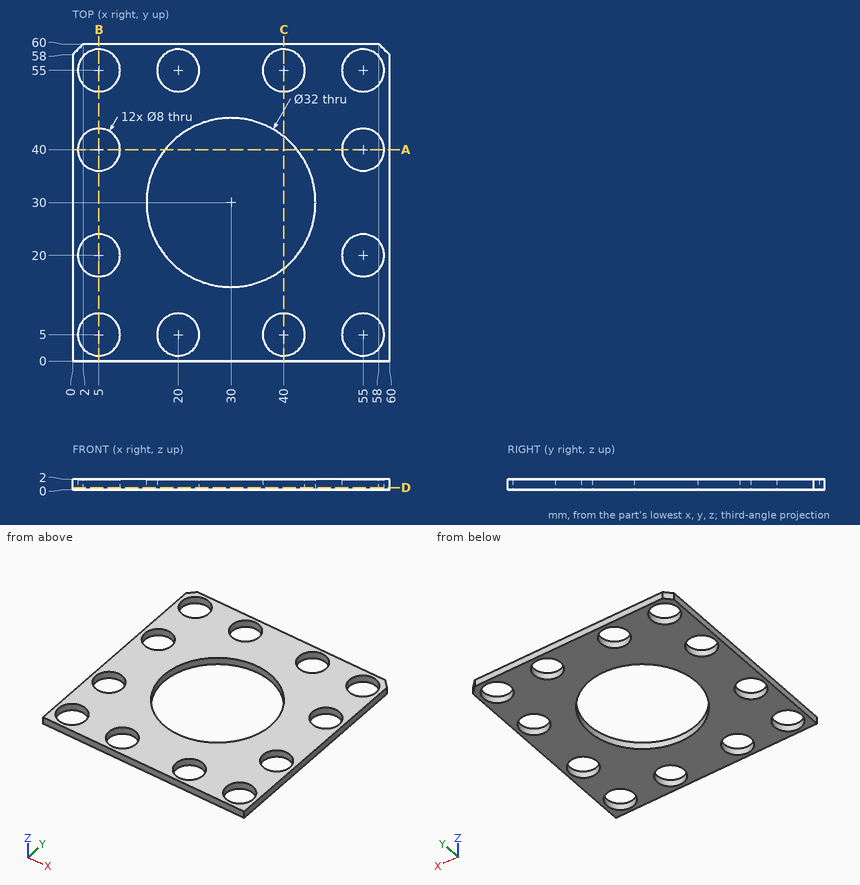
Study the drawing (mm; zero at the part's minimum x, y, z) and answer. Round coordinates to 2 decimals unless told otherwise and drop trailing zeros. Loops run counter-clockwise (first coordinate to the right, second up) from the corner with the lowest first, then second, coordinate; pieces in that order, holes last. Notation, with made-up numbers: (32.5, -1.5) -> (50.5, -1.5) arc R18 cw to (50.5, 23.5) -> close; hole circle Ø2 at (-31, 30.5). An arc over 180 degrees is marked (long way). Write each question's results on one line, items separated by ' | '. Start each with the question number.
1. Section A-A (y = 40) is taken. Determine the outline of the cut face in (x, z).
2. Section D-D (z = 0.35) is taken. State how many separate pieces and enclosed holes the cut face has, plus the area to 3 significant figures.
3. Given pin 1 Ø5 at (x, y) = (40, 5) entering from -Z, flat-ended and moving along its own axis, determine where the tip first touches the part or whether it passes through.
4. Find the intervals of material crossed by probe 1 along Y at (x, z) = (55, 1.25); probe 2 along Y at (x, z) = (21.5, 0.95); probe 3 along Y at (x, z) = (8, 1.25), in increasing order. Write a range as from..to.
5. Section B-B (x = 5) is taken. Determine the outline of the cut face in (y, z).
Evaluation:
1) outline: (0, 0) -> (1, 0) -> (1, 2) -> (0, 2) -> close; (9, 0) -> (17.51, 0) -> (17.51, 2) -> (9, 2) -> close; (42.49, 0) -> (51, 0) -> (51, 2) -> (42.49, 2) -> close; (59, 0) -> (60, 0) -> (60, 2) -> (59, 2) -> close
2) separate pieces: 1 | enclosed holes: 13 | area: 2,190 mm2
3) pin 1: passes through
4) probe 1: y = 0..1, 9..16, 24..36, 44..51, 59..60 | probe 2: y = 0..1.29, 8.71..16.44, 43.56..51.29, 58.71..60 | probe 3: y = 0..2.35, 7.65..17.35, 22.65..37.35, 42.65..52.35, 57.65..60
5) outline: (0, 0) -> (1, 0) -> (1, 2) -> (0, 2) -> close; (9, 0) -> (16, 0) -> (16, 2) -> (9, 2) -> close; (24, 0) -> (36, 0) -> (36, 2) -> (24, 2) -> close; (44, 0) -> (51, 0) -> (51, 2) -> (44, 2) -> close; (59, 0) -> (60, 0) -> (60, 2) -> (59, 2) -> close
